For this review, take the finished solid that the model builds, in its own axes (mm). Give positions to 0.01 mm unless a question says otherwise; leave off trailing zeros. Loops run counter-clockwise (first coordinate to the right, second up) from the corner with the lowest first, then second, coordinate; pieces in that order, holes last. Notation, with made-up numbers: (-17.75, 76) - (16.25, 76) arc R13 ccw to (16.25, 81) - close; hole circle Ø4 at (40, 85). An arc over 180 degrees is marked (long way). Put each result on its own line as item: value. Start each with the question number.
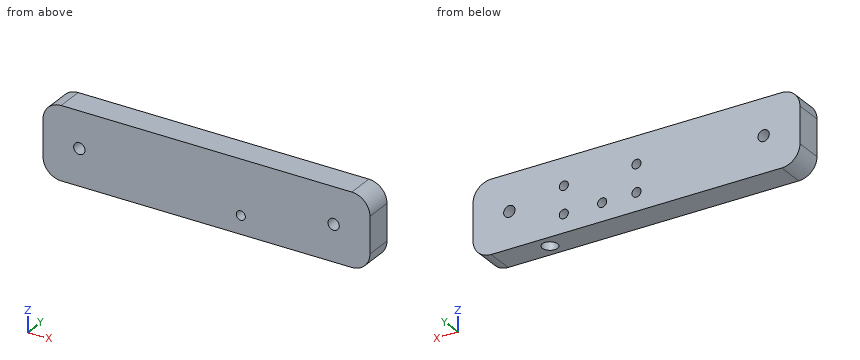
from build123d import *

# Parameters (mm, degrees)
F0_W      = 228.6
F0_H      = 50.8
F1_DEPTH  = 19.05
F2_D      = 7.9375
F3_R      = 12.7
F4_D      = 6.35
F4_DEPTH  = 12.7
F4_TIP    = 1.9077324654
F9_D      = 6.35
F10_R     = 12.7
F12_D     = 10.71626
F12_DEPTH = 12.7
F12_TIP   = 3.2194893086


with BuildPart() as f1:
    # F0 (on Front) → F1 (new body)
    with BuildSketch(Plane.XZ):
        with Locations((-114.3, 25.4)):
            Rectangle(F0_W, F0_H)
    extrude(amount=F1_DEPTH)

    # F2 (through all)
    with Locations(Plane(origin=(0, 0, 0), x_dir=(1, 0, 0), z_dir=(0, 1, 0))):
        with Locations((-203.2, -25.4), (-25.4, -25.4)):
            Hole(F2_D / 2)

    # F3
    f3_edges = [f1.edges().sort_by_distance(p)[0] for p in [
        (0, -9.525, 0),
        (0, -9.525, 50.8),
    ]]
    fillet(f3_edges, radius=F3_R)

    # F4
    with Locations(Plane(origin=(0, 0, 0), x_dir=(1, 0, 0), z_dir=(0, 1, 0))):
        with Locations((-114.3, -31.75), (-114.3, -12.7), (-63.5, -12.7), (-63.5, -31.75)):
            Hole(F4_D / 2, depth=F4_DEPTH)
            with Locations((0, 0, -(F4_DEPTH + F4_TIP / 2))):  # 118° drill point
                Cone(0, F4_D / 2, F4_TIP, mode=Mode.SUBTRACT)


with BuildPart() as f5_1:
    # F5: instance of F1
    add(f1.part.mirror(Plane(origin=(-114.9742152146, -19.05, 25.4), x_dir=(1, 0, 0), z_dir=(0, -1, 0))))


with BuildPart() as f7_1:
    # F7: instance of F5_1
    add(f5_1.part.mirror(Plane(origin=(-114.9742152146, -19.05, 25.4), x_dir=(-1, 0, 0), z_dir=(0, 1, 0))))

    # F9 (through all)
    with Locations(Plane(origin=(0, 0, 0), x_dir=(1, 0, 0), z_dir=(0, 1, 0))):
        with Locations((-90.297, -12.7)):
            Hole(F9_D / 2)

    # F10
    f10_edges = [f7_1.edges().sort_by_distance(p)[0] for p in [
        (-228.6, -9.525, 50.8),
        (-228.6, -9.525, 0),
    ]]
    fillet(f10_edges, radius=F10_R)

    # F12
    with Locations(Plane(origin=(0, 0, 0), x_dir=(1, 0, 0), z_dir=(0, 0, -1))):
        with Locations((-47.8227784872, 9.525)):
            Hole(F12_D / 2, depth=F12_DEPTH)
            with Locations((0, 0, -(F12_DEPTH + F12_TIP / 2))):  # 118° drill point
                Cone(0, F12_D / 2, F12_TIP, mode=Mode.SUBTRACT)


solid = f7_1.part
1) Insertion check: P1, Ø5.5, axis at x = -114.3, z = 31.75, coming from the +Y side; P2, Ø6.5, axis at x = -47.82, y = -9.52, coming from the -Z side. Each pin has a flat end and moves straight along its axis. Give the tip position at first contact, or say it passes through.
2) Take a section at B-B on x = -203.2. State the section outline as (y, z) points, and give its area (3 significant figures).
3) Take a section at A-A on z = 25.4. State the section outline as (x, y) points.
4) Wall thickness on probe 1 along Z at (x, y) = (-63.5, -8.75) (3 decimals); probe 2 along X at (y, z) = (-4, 25.4); probe 3 along X at (y, z) = (-5.75, 31.5): over which ranges is each line inside the solid? List them lowest first.
Answers follow:
1. P1: y = -12.96
1. P2: z = 13.96
2. outline: (-19.05, 0) - (0, 0) - (0, 21.43) - (-19.05, 21.43) - close; (-19.05, 29.37) - (0, 29.37) - (0, 50.8) - (-19.05, 50.8) - close
2. area: 817 mm2
3. outline: (-228.6, -19.05) - (-207.17, -19.05) - (-207.17, 0) - (-228.6, 0) - close; (-199.23, -19.05) - (-29.37, -19.05) - (-29.37, 0) - (-199.23, 0) - close; (-21.43, -19.05) - (0, -19.05) - (0, 0) - (-21.43, 0) - close
4. probe 1: 0 to 9.525, 15.875 to 28.575, 34.925 to 50.8
4. probe 2: -228.6 to -207.17, -199.23 to -29.37, -21.43 to 0
4. probe 3: -228.6 to -117.47, -111.13 to -66.67, -60.33 to 0
